from build123d import *

# Parameters (mm, degrees)
F0_R     = 4
F1_DEPTH = 4
F2_R     = 6.99999


# Not quite as in the source:
# - a fillet or chamfer is up to 0.001 mm smaller than in the source, because OpenCascade refuses the exact size
# - a feature names something its author has since deleted; it is built from what else it names


with BuildPart() as f1:
    # F0 (on Front) → F1 (new body)
    with BuildSketch(Plane.XZ):
        Polygon((7, 57), (-7, 57), (-7, 7), (-57, 7), (-57, -7), (57, -7), (57, 7), (7, 7), align=None)
        with Locations((-50, 0)):
            Circle(F0_R, mode=Mode.SUBTRACT)
        Circle(F0_R, mode=Mode.SUBTRACT)
        with Locations((50, 0)):
            Circle(F0_R, mode=Mode.SUBTRACT)
        with Locations((0, 50)):
            Circle(F0_R, mode=Mode.SUBTRACT)
    extrude(amount=F1_DEPTH)

    # F2 (radius 7 in the source; OpenCascade refuses exactly that, so slightly less here)
    f2_edges = [f1.edges().sort_by_distance(p)[0] for p in [
        (57, -2, -7),
        (57, -2, 7),
        (7, -2, 57),
        (-7, -2, 57),
        (-57, -2, 7),
        (-57, -2, -7),
    ]]
    fillet(f2_edges, radius=F2_R)


solid = f1.part
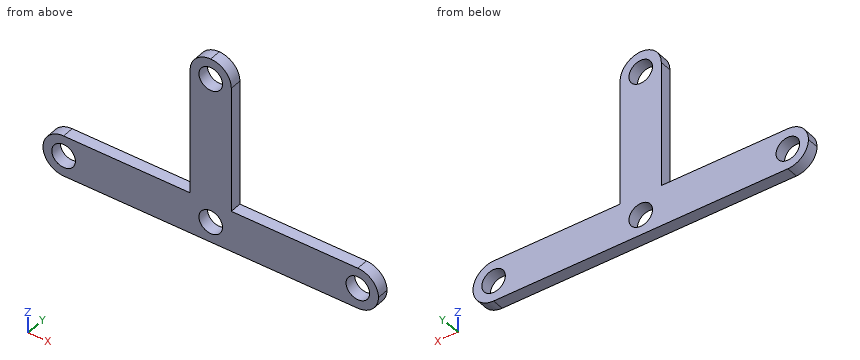
The listing builds one solid part. Answer for the finished solid, in the listing's coordinates (mm). Give positions to 0.01 mm unless a question says otherwise; leave off trailing zeros. Loops run counter-clockwise (first coordinate to the right, second up) from the corner with the lowest first, then second, coordinate; pieces in that order, holes last. Notation, with made-up numbers: (44.5, 45.25) - (71.5, 45.25) arc R16 ccw to (71.5, 54.25) - close; hole circle Ø3 at (-21.5, 79.5). An arc over 180 degrees is marked (long way). Answer as a JSON object with one key per item and string values.
1. A cutting plane is placed at B-B (z = 41). Write down the section's boundary in (x, y), then the cut area to 3 significant figures.
Determined:
{"outline": "(-7, -4) - (7, -4) - (7, 0) - (-7, 0) - close", "area": "56.0 mm²"}
2. Flat-ended cylindrical pins translate along their axes: pin 1 Ø2 at (x, y) = (-28.5, -3) entering from +Z; pin 2 Ø1 at (y, z) = (-3.5, 16.5) entering from +X; pin 3 Ø10.5 at (x, z) = (0, 0) entering from +Y. Find the tip coordinate at first contact, or state that the pin passes through.
Determined:
{"pin 1": "z = 7", "pin 2": "x = 7", "pin 3": "y = 0"}
3. Find the intervals of material crossed by L1, parallel to Z at x = 0, y = -1.2; L2, parallel to Z at x = -50, y = -1.85; L3, parallel to X at y = -2.25, z = 12.5, in increasing order. Write a range as [from, to].
Determined:
{"L1": "[-7, -4], [4, 46], [54, 57]", "L2": "[-7, -4], [4, 7]", "L3": "[-7, 7]"}
4. A cutting plane is placed at A-A (y = -2.8). Give the number of separate pieces and of enclosed holes in the cut face, then the cut area to 3 significant figures.
Determined:
{"separate pieces": "1", "enclosed holes": "4", "area": "2,030 mm²"}
5. A cutting plane is placed at C-C (x = 11.5). Write down the section's boundary in (y, z), then the cut area to 3 significant figures.
Determined:
{"outline": "(-4, -7) - (0, -7) - (0, 7) - (-4, 7) - close", "area": "56.0 mm²"}
